Job drawing, mm, ordinate dimensions from the low corner. One solid piece. A direction names the side the tool comes from. Give positions to 0.01 mm unless a question says otherwise; leave off trailing zeros. Write each loop counter-clockwise with the first axis right and the second up, starting at its lowest first coordinate (ties: lowest second). Pieces come first, ordered by that corner, then holes. Notation, with made-up numbers: M 70.25,-31 L 81.25,-31 A23 cw 81.25,-2 Z; hole C -9,3 d7. An arc over 180 degrees is marked long. Answer as CSV lines item,"result". Start each with the question number.
1) Slice it at C-C, the plane y = 10. Give the cut face in (x, z), plus the area to 3 significant figures.
2) Slice it at B-B, the plane z = 4. Give the cut face in (x, y), plus the area to 3 significant figures.
3) Pin check, flat tips, straight feed: pin 1 Ø0.8 at (x, z) = (22, 21.5) entering from +Y; pin 2 Ø4 at (y, z) = (46, 21) entering from -X; pin 3 Ø9 at (x, y) = (8, 12) entering from +Z; pin 4 Ø5.5 at (x, y) = (32, 10) entering from -Z. Stop position of each tip, or through.
4) Tool access for the marked faces 1, 2, 3 and 4: list every direction of +Z, -Z, +X, -X, +Y, -Y with a clear straight run to the whole face (end or side of a thin tool).
5) Slice it at A-A, the plane x = 8. Give the cut face in (y, z).
6) Mould opens along Y. For the marked faces 5, 6, 7 and 8 say: pulls with the +Y half, pulls with the -Y half, needs draft (parallel to the pull), parting line crosses it, or undercut.
7) Slice it at D-D, the plane y = 32. Give the cut face in (x, z), plus the area to 3 significant figures.
8) Wall check: line 1 along X through (y, z) = (31, 13.75); line 2 along Y through (x, z) = (32, 11.25); line 3 along X through (y, z) = (42.5, 18.5). Give the ranges that are in metal, low to high. Write a range as from..to.
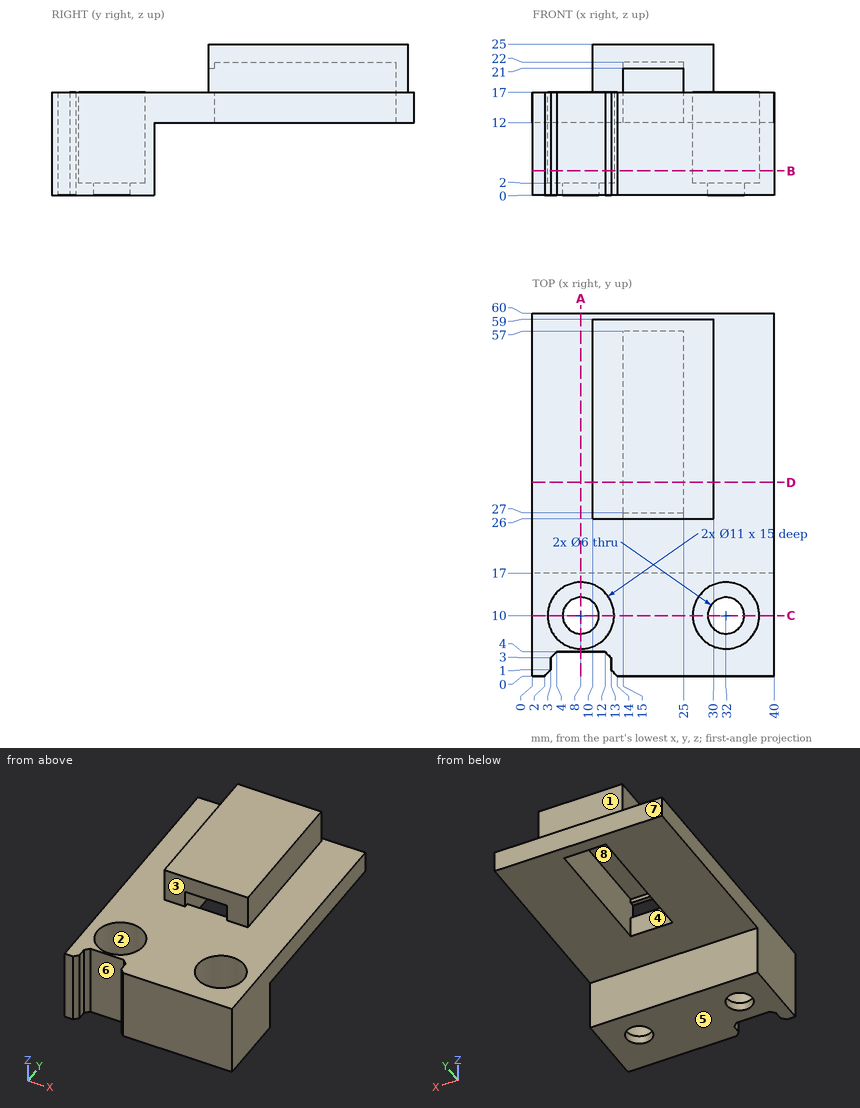
Found:
1,outline,"M 0,0 L 5,0 L 5,2 L 2.5,2 L 2.5,17 L 0,17 Z; M 11,0 L 29,0 L 29,2 L 26.5,2 L 26.5,17 L 13.5,17 L 13.5,2 L 11,2 Z; M 35,0 L 40,0 L 40,17 L 37.5,17 L 37.5,2 L 35,2 Z"
1,area,"326 mm²"
2,outline,"M 0,0 L 2,0 L 3,1 L 3,3 L 4,4 L 12,4 L 13,3 L 13,1 L 14,0 L 40,0 L 40,17 L 0,17 Z; hole C 8,10 d11; hole C 32,10 d11"
2,area,"450 mm²"
3,pin 1,"y = 59"
3,pin 2,"x = 10"
3,pin 3,"z = 17"
3,pin 4,"through"
4,face 1,"+Z, +X, -X, +Y"
4,face 2,"+Z"
4,face 3,"+Z, +X, -X, -Y"
4,face 4,"-Z"
5,outline,"M 4,0 L 7,0 L 7,2 L 4.5,2 L 4.5,17 L 4,17 Z; M 13,0 L 17,0 L 17,12 L 60,12 L 60,17 L 15.5,17 L 15.5,2 L 13,2 Z"
6,face 5,"needs draft"
6,face 6,"pulls with the -Y half"
6,face 7,"pulls with the +Y half"
6,face 8,"undercut"
7,outline,"M 0,12 L 15,12 L 15,22 L 25,22 L 25,12 L 40,12 L 40,17 L 30,17 L 30,25 L 10,25 L 10,17 L 0,17 Z"
7,area,"260 mm²"
8,line 1,"0..15, 25..40"
8,line 2,"0..4.5, 15.5..17"
8,line 3,"10..15, 25..30"
